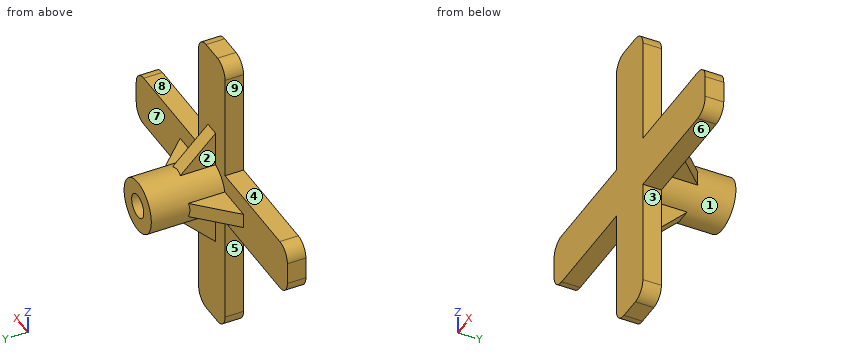
from build123d import *

# Parameters (mm, degrees)
BOSS_EXTRUDE1_DEPTH = 3.175
SKETCH2_R           = 4.572
SKETCH2_R_2         = 2.032
BOSS_EXTRUDE2_DEPTH = 12.7
BOSS_EXTRUDE3_DEPTH = 1.27
BOSS_EXTRUDE4_DEPTH = 1.27


with BuildPart() as part:
    # Sketch1 → Boss-Extrude1 (new body)
    with BuildSketch(Plane(origin=(0, 0, 0), x_dir=(1, 0, 0), z_dir=(0, 1, 0))):
        with BuildLine():
            Line((-25.4, 1.905), (-25.4, -1.905))
            ThreePointArc((-25.4, -1.905), (-24.656051224, -3.701051224), (-22.86, -4.445))
            Line((-22.86, -4.445), (-4.445, -4.445))
            Line((-4.445, -4.445), (-4.445, -22.86))
            ThreePointArc((-4.445, -22.86), (-3.701051224, -24.656051224), (-1.905, -25.4))
            Line((-1.905, -25.4), (1.905, -25.4))
            ThreePointArc((1.905, -25.4), (3.701051224, -24.656051224), (4.445, -22.86))
            Line((4.445, -22.86), (4.445, -4.445))
            Line((4.445, -4.445), (22.86, -4.445))
            ThreePointArc((22.86, -4.445), (24.656051224, -3.701051224), (25.4, -1.905))
            Line((25.4, -1.905), (25.4, 1.905))
            ThreePointArc((25.4, 1.905), (24.656051224, 3.701051224), (22.86, 4.445))
            Line((22.86, 4.445), (4.445, 4.445))
            Line((4.445, 4.445), (4.445, 22.86))
            ThreePointArc((4.445, 22.86), (3.701051224, 24.656051224), (1.905, 25.4))
            Line((1.905, 25.4), (-1.905, 25.4))
            ThreePointArc((-1.905, 25.4), (-3.701051224, 24.656051224), (-4.445, 22.86))
            Line((-4.445, 22.86), (-4.445, 4.445))
            Line((-4.445, 4.445), (-22.86, 4.445))
            ThreePointArc((-22.86, 4.445), (-24.656051224, 3.701051224), (-25.4, 1.905))
        make_face()
    extrude(amount=BOSS_EXTRUDE1_DEPTH)

    # Sketch2 → Boss-Extrude2 (add)
    with BuildSketch(Plane(origin=(0, 3.175, 0), x_dir=(1, 0, 0), z_dir=(0, 1, 0))):
        with Locations(Location((0, 0, 0), (0, 0, 90))):
            Circle(SKETCH2_R)
        with Locations(Location((0, 0, 0), (0, 0, 270))):
            Circle(SKETCH2_R_2, mode=Mode.SUBTRACT)
    extrude(amount=BOSS_EXTRUDE2_DEPTH)

    # Sketch9 → Boss-Extrude3 (add, symmetric)
    with BuildSketch(Plane.XY):
        Polygon((-10.659295588, 3.175), (-4.309295588, 3.175), (-4.309295588, 9.525), align=None)
        Polygon((10.659295588, 3.175), (4.309295588, 3.175), (4.309295588, 9.525), align=None)
    extrude(amount=BOSS_EXTRUDE3_DEPTH, both=True)

    # Sketch10 → Boss-Extrude4 (add, symmetric)
    with BuildSketch(Plane(origin=(0, 0, 0), x_dir=(0, 0, -1), z_dir=(1, 0, 0))):
        Polygon((-10.456553942, 3.175), (-4.106553942, 3.175), (-4.106553942, 9.525), align=None)
        Polygon((4.106553942, 9.525), (10.456553942, 3.175), (4.106553942, 3.175), align=None)
    extrude(amount=BOSS_EXTRUDE4_DEPTH, both=True)


solid = part.part
For this review, take the finished solid that the model builds, in its own axes (mm). Face numbers are marked on the shaded views. A direction names the side the tool comes from. Give positions to 0.01 mm unless a question says otherwise; leave off trailing zeros. Order: outer loops, then holes, each group sorted by start corner. A loop starts at its lowest first (then second) coordinate and runs counter-clockwise, first axis right, second up. Notation, with made-up numbers: M 42.25,43.25 L 71.25,43.25 A13 cw 71.25,67.25 Z; hole C 73.5,-7.75 d1. An arc over 180 degrees is marked long. Answer in a Markdown table with one row per item. Add a question column.
(1) For pin 1 (7 mm diameter, centred on x = 8.5, y = 6, fed in from +Z) (3 decimals); pin 2 (2 mm diameter, centred on y = 7.5, z = 7.5, fed in from +X); pin 3 (2.5 mm diameter, centred on y = 1, z = -11.5, fed in from -X) (3 decimals), all flat-tipped, find the tip position at first contact; note any pin that passes through.
(2) Mouldability with a two-part tool opening along X and no side actions: class the marked faces 1, 2, 3 and 4 as +X half, -X half, draft (parallel to the pull), parting line (faces both ways), or undercut.
(3) Consider section A-A on y = 10.5. State the section outline as (x, z) points.
(4) Consider section D-D on z = 6.5. State the section outline as (x, y) points (3 decimals).
(5) Wall thickness on probe 1 along X at (y, z) = (13, 0); probe 2 along Y at (x, z) = (-12, -4) (3 decimals); probe 3 along Z at (x, y) = (-11, 2) (3 decimals): over which ranges is each line inside the solid? List them lowest first. Write a range as [from, to].
(6) For the marked faces 5, 6, 7, 8 and 9, list the 3-axis set-ups (+Z, -Z, +X, -X, +Y, -Y) from which the entire face can be reached by the end or side of a thin tool; tool diameter is ignored.
(7) Consider section C-C on z = -6. State the section outline as (x, y) points (3 decimals).
(8) Consider section B-B on x = 0. State the section outline as (y, z) points (3 decimals), and give its area (3 significant figures).
Evaluation:
| question | item | result |
|---|---|---|
| 1 | pin 1 | stops at z = 4.445 |
| 1 | pin 2 | stops at x = 1.27 |
| 1 | pin 3 | stops at x = -4.445 |
| 2 | face 1 | parting line |
| 2 | face 2 | -X half |
| 2 | face 3 | +X half |
| 2 | face 4 | draft |
| 3 | outline | C 0,0 d9.14; hole C 0,0 d4.06 |
| 4 | outline | M -4.445,0 L 4.445,0 L 4.445,3.175 L 1.27,3.175 L 1.27,7.132 L -1.27,7.132 L -1.27,3.175 L -4.445,3.175 Z |
| 5 | probe 1 | x = [-4.57, -2.03], [2.03, 4.57] |
| 5 | probe 2 | y = [0, 3.175] |
| 5 | probe 3 | z = [-4.445, 4.445] |
| 6 | face 5 | -Z, -X, +Y, -Y |
| 6 | face 6 | -Z, +X, +Y, -Y |
| 6 | face 7 | +Y |
| 6 | face 8 | +Z, +X, +Y, -Y |
| 6 | face 9 | +Z, -X, +Y, -Y |
| 7 | outline | M -4.445,0 L 4.445,0 L 4.445,3.175 L 1.27,3.175 L 1.27,7.632 L -1.27,7.632 L -1.27,3.175 L -4.445,3.175 Z |
| 8 | outline | M 0,-25.4 L 3.175,-25.4 L 3.175,-10.457 L 9.06,-4.572 L 15.875,-4.572 L 15.875,-2.032 L 3.175,-2.032 L 3.175,2.032 L 15.875,2.032 L 15.875,4.572 L 9.06,4.572 L 3.175,10.457 L 3.175,25.4 L 0,25.4 Z |
| 8 | area | 260 mm^2 |
